The listing builds one solid part. Answer for the finished solid, in the listing's coordinates (mm). A direction names the side the tool comes from. Round coordinates to 2 decimals unless told otherwise and drop trailing zeros. Return JSON: item names as keys, results as strings. Group by question number.
(1) Consider line 1 (Y direction, x = -7.5, z = 3); line 2 (Y direction, x = 0, z = 5); line 3 (Y direction, x = 5, z = 3.25). Determine where each line is inside the solid, lowest interval first. Write a range as [from, to].
(2) Which of the six approach directions +Z, -Z, +X, -X, +Y, -Y give full straight-line access (tool end or side, diameter ignored) to faces 1 (the face through (0, 102, 0)), 2 (the face through (0, 80, -6)), 3 (the face through (-1.6, 93, 5))?
(3) Each of these flat-tipped pins is pushed along its axis until it touches: pin 1 (1.5 mm diameter, centred on x = -6.5, z = 5, fed in from -Y); pin 2 (5 mm diameter, centred on x = -3, y = 43.5, fed in from -Z); pin 3 (5 mm diameter, centred on x = 4, z = -2.5, fed in from -Y). Where does it stop, or does it pass through?
Autodesk Inventor part; units mm, degrees
ref_plane "YZ Plane" through (0, 0, 0) normal (1, 0, 0) x (0, 1, 0)
ref_plane "XZ Plane" through (0, 0, 0) normal (0, 1, 0) x (-1, 0, 0)
ref_plane "XY Plane" through (0, 0, 0) normal (0, 0, 1) x (1, 0, 0)
sketch "Sketch1" plane through (0, 0, 0) normal (1, 0, 0) x (0, 1, 0)
  line L0 (0, 0) -> (104.5, 0)
  line L1 (0, 0) -> (75, 0)
  line L2 (75, 0) -> (75, 3)
  line L3 (75, 3) -> (0, 3)
  line L4 (0, 3) -> (0, 0)
  line L5 (75, 0) -> (85, 0)
  line L6 (85, 0) -> (85, 6)
  line L7 (85, 6) -> (75, 6)
  line L8 (75, 6) -> (75, 0)
  line L9 (85, 0) -> (87, 0)
  line L10 (87, 0) -> (87, 5.25)
  line L11 (87, 5.25) -> (85, 5.25)
  line L12 (85, 5.25) -> (85, 0)
  line L13 (87, 0) -> (90, 0)
  line L14 (90, 0) -> (90, 9)
  line L15 (90, 9) -> (87, 9)
  line L16 (87, 9) -> (87, 0)
  line L17 (90, 0) -> (96, 0)
  line L18 (96, 0) -> (96, 5.25)
  line L19 (96, 5.25) -> (90, 5.25)
  line L20 (90, 5.25) -> (90, 0)
  line L21 (96, 0) -> (102, 0)
  line L22 (102, 0) -> (102, 9)
  line L23 (102, 9) -> (96, 9)
  line L24 (96, 9) -> (96, 0)
  point P0 (102, 2.5)
  dimension "d0" = 6
  dimension "d2" = 12
  dimension "d3" = 10
  dimension "d5" = 2
  dimension "d6" = 75
  dimension "d7" = 10.5
  dimension "d8" = 18
  dimension "d9" = 3
  dimension "d10" = 6
  dimension "d11" = 6
revolve "Revolution1" add sketch "Sketch1" angle 360 about axis through (0, 0, 0) along (0, 1, 0)
chamfer "Chamfer1" distance 1 angle 45 1 edges at (0, 0, -3)
chamfer "Chamfer2" distance 1 angle 45 1 edges at (0, 75, -6)
chamfer "Chamfer4" distance 0.5 angle 45 2 edges at (0, 102, -9) (0, 96, -9)
fillet "Fillet1" radius 2 2 edges at (0, 90, -5.25) (0, 96, -5.25)
thread "Thread1"
properties part number "05_Que_tham_dau"
Answer below:
{
 "1": {"line 1": "y = [87, 90], [96, 102]", "line 2": "y = [75, 102]", "line 3": "y = [75.96, 85], [87, 90.47], [95.53, 102]"},
 "2": {"face 1": "+Z, -Z, +X, -X, +Y", "face 2": "-Y", "face 3": "none"},
 "3": {"pin 1": "stops at y = 87", "pin 2": "stops at z = -2.96", "pin 3": "stops at y = 0.22"}
}
